Part print with two shaded views. Sizes in mm from the minimum x, y, z corner. A direction names the side the tool comes from. Coordinates: 2 decimals unless noted, no trailing zeros. Write each loop counter-clockwise with the first axis right and the second up, starting at its lowest first coordinate (ties: lowest second). Pieces come first, ordered by that corner, then holes. Notation, with made-up numbers: M 27,82.5 L 85,82.5 A20 cw 85,105.5 Z; hole C 31,71 d4. An arc over 180 degrees is marked long. One line per question, with ' | ' between items. Start each with the question number.
(1) Cut at D-D (z = 1). Write the cut outline in (x, y), plus the area to 3 significant figures.
(2) Tool access for the marked faces 1 and 2: list every direction of +Z, -Z, +X, -X, +Y, -Y with a clear straight run to the whole face (end or side of a thin tool).
(3) Wall check: probe 1 along X at (y, z) = (0.5, 6.5); probe 2 along Z at (x, y) = (23.75, 2.25); probe 3 along X at (y, z) = (5.25, 1). Give the ranges that are in metal, low to high.
(4) Two-plate mould, pull along X, no slides. Class the marked faces 3, 4 and 5: +X half, -X half, draft (parallel to the pull), parting line (faces both ways), or undercut.
(5) Flat gauge pins, fed straight in: pin 1 Ø4 at (y, z) = (9, 5.5) entering from -X; pin 2 Ø4.5 at (x, y) = (12.5, 4) entering from -Z. Where does each tip first touch, or does it go through?
(6) Cut at A-A (z = 10.5). Write the cut outline in (x, y).
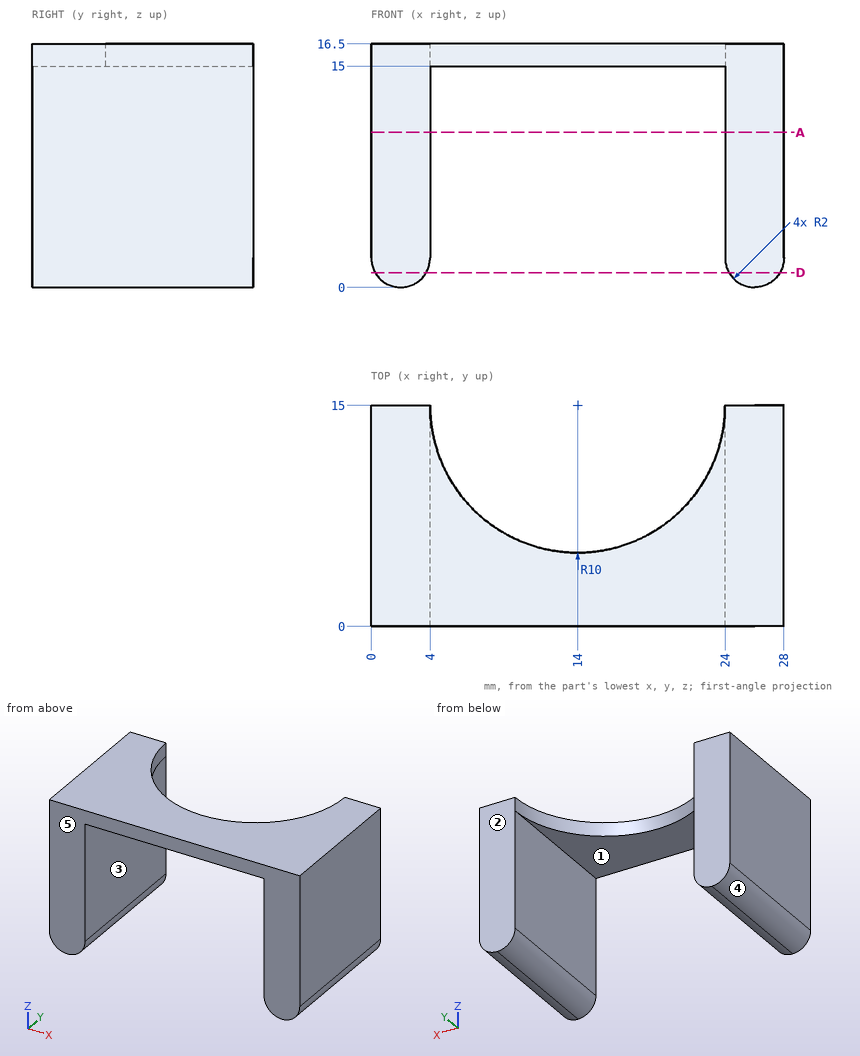
Filled in:
1) outline: M 0.27,0 L 3.73,0 L 3.73,15 L 0.27,15 Z; M 24.27,0 L 27.73,0 L 27.73,15 L 24.27,15 Z | area: 104 mm²
2) face 1: -Z, +Y, -Y | face 2: +Z, -Z, +X, -X, +Y
3) probe 1: 0 to 4, 24 to 28 | probe 2: 15 to 16.5 | probe 3: 0.27 to 3.73, 24.27 to 27.73
4) face 3: undercut | face 4: -X half | face 5: draft
5) pin 1: x = 0 | pin 2: z = 15
6) outline: M 0,0 L 4,0 L 4,15 L 0,15 Z; M 24,0 L 28,0 L 28,15 L 24,15 Z
